```python
from build123d import *

# Parameters (mm, degrees)
SKETCH1_R           = 2.5
BOSS_EXTRUDE1_DEPTH = 6
FILLET1_R           = 4


with BuildPart() as part:
    # Sketch1 → Boss-Extrude1 (new body)
    with BuildSketch(Plane(origin=(0, 0, 0), x_dir=(1, 0, 0), z_dir=(0, 1, 0))):
        Polygon((-4, 14.999990394), (-4, 8.999990394), (-12, 8.999990394), (-12, 2.999990394), (-4, 2.999990394), (-4, -3.000009606), (-12, -3.000009606), (-12, -9.000009606), (-4, -9.000009606), (-4, -15.000009606), (4, -15.000009606), (4, 14.999990394), align=None)
        with Locations(Location((0, 5.5, 0), (0, 0, 270))):
            Circle(SKETCH1_R, mode=Mode.SUBTRACT)
        with Locations(Location((0, -5.5, 0), (0, 0, 270))):
            Circle(SKETCH1_R, mode=Mode.SUBTRACT)
    extrude(amount=BOSS_EXTRUDE1_DEPTH)

    # Fillet1
    fillet1_edges = [part.edges().sort_by_distance(p)[0] for p in [
        (-4, 3, 15.000009606),
        (-4, 3, -14.999990394),
        (4, 3, 15.000009606),
        (4, 3, -14.999990394),
    ]]
    fillet(fillet1_edges, radius=FILLET1_R - 0.0001)  # a hair under: the kernel refuses the full size


solid = part.part
```
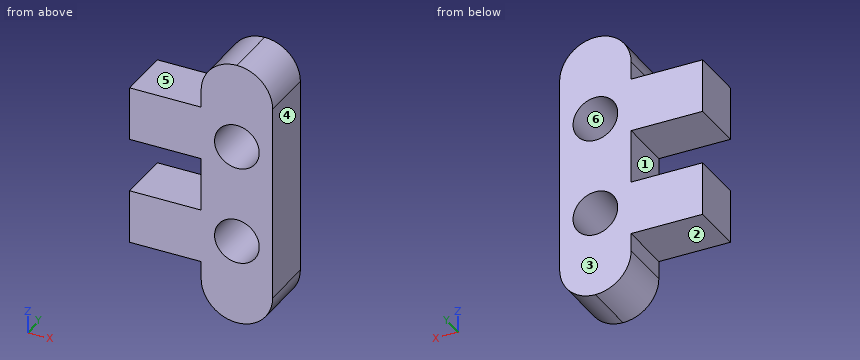
Geometry check sheet. Reference: the model listing, model coordinates, mm. Face numbers are marked on the shaded views. A direction names the side the tool comes from. Give positions to 0.01 mm unless a question says otherwise; leave off trailing zeros. Write each loop counter-clockwise with the first axis right and the second up, starting at its lowest first coordinate (ties: lowest second). Pieces come first, ordered by that corner, then holes. Notation, with made-up numbers: (30, 17.5) - (64, 17.5) arc R25 ccw to (64, 39.5) - close; hole circle Ø6 at (27, 4.25). An arc over 180 degrees is marked (long way). Use a Markdown table: item, result.
Q1. Section check B-B, the plane x = -9.75. Enter the section's corners in (y, z).
Computed:
| item | result |
|---|---|
| outline | (0, -9) - (6, -9) - (6, -3) - (0, -3) - close; (0, 3) - (6, 3) - (6, 9) - (0, 9) - close |
Q2. Go/stop test with flat-tipped pins: P1, Ø2, axis at y = 3, z = 11.5, coming from the -X side; P2, Ø4.5, axis at x = 0, z = -5.5, coming from the -Y side; P3, Ø3, axis at x = -6.5, y = 1.5, coming from the -Z side; P4, Ø1, axis at x = -6, y = 2.5, coming from the +Z side. Record where each tip stops, or that it passes through.
Computed:
| item | result |
|---|---|
| P1 | stops at x = -4 |
| P2 | passes through |
| P3 | stops at z = -9 |
| P4 | stops at z = 9 |
Q3. Draft check along Z on the marked faces 4, 5 and 6. Enter one of: pulls with the +Z half, pulls with the -Z half, needs draft (parallel to the pull), parting line crosses it, or undercut.
Computed:
| item | result |
|---|---|
| face 4 | needs draft |
| face 5 | pulls with the +Z half |
| face 6 | undercut |
Q4. Section check D-D, the plane x = 1. Enter the section's corners in (y, z).
Computed:
| item | result |
|---|---|
| outline | (0, -14.87) - (6, -14.87) - (6, -7.79) - (0, -7.79) - close; (0, -3.21) - (6, -3.21) - (6, 3.21) - (0, 3.21) - close; (0, 7.79) - (6, 7.79) - (6, 14.87) - (0, 14.87) - close |
Q5. Thickness scan on L1, parallel to Z at x = -8.5, y = 5.75; L2, parallel to X at y = 1.75, z = 5.5; L3, parallel to Z at x = -1.5, y = 5.7. Record the ranges inside material, lowest first. Write a range as [from, to].
Computed:
| item | result |
|---|---|
| L1 | z = [-9, -3], [3, 9] |
| L2 | x = [-12, -2.5], [2.5, 4] |
| L3 | z = [-14.71, -7.5], [-3.5, 3.5], [7.5, 14.71] |
Q6. Section check A-A, the plane z = -5.5. Enter the section's corners in (x, y).
Computed:
| item | result |
|---|---|
| outline | (-12, 0) - (-2.5, 0) - (-2.5, 6) - (-12, 6) - close; (2.5, 0) - (4, 0) - (4, 6) - (2.5, 6) - close |
Q7. Section check C-C, the plane y = 2.95. Give the number of separate pieces and of enclosed holes in the cut face, then the cut area to 3 significant figures.
Computed:
| item | result |
|---|---|
| separate pieces | 1 |
| enclosed holes | 2 |
| area | 283 mm² |
Q8. Set-up check for the marked faces 1, 2 and 3: record each of +Z, -Z, +X, -X, +Y, -Y from which the full face is reachable in a straight line by a thin tool's end or side.
Computed:
| item | result |
|---|---|
| face 1 | -X, +Y, -Y |
| face 2 | -Z, -X, +Y, -Y |
| face 3 | +Z, -Z, +X, -X, +Y |
